from build123d import *

# Parameters (mm, degrees)
SKETCH1_W           = 12.7
SKETCH1_H           = 16.891
BOSS_EXTRUDE1_DEPTH = 3.175
SKETCH2_R           = 2.54
CUT_EXTRUDE1_DEPTH  = 4.175
SKETCH3_W           = 12.7
SKETCH3_H           = 3.175
BOSS_EXTRUDE2_DEPTH = 22.225
SKETCH4_R           = 2.54
CUT_EXTRUDE2_DEPTH  = 4.175
CUT_EXTRUDE3_DEPTH  = 4.175
CUT_EXTRUDE4_DEPTH  = 4.175


with BuildPart() as part:
    # Sketch1 → Boss-Extrude1 (new body)
    with BuildSketch(Plane(origin=(0, 0, 0), x_dir=(1, 0, 0), z_dir=(0, 1, 0))):
        with Locations((-16.427296288, 6.362973118)):
            Rectangle(SKETCH1_W, SKETCH1_H)
    extrude(amount=BOSS_EXTRUDE1_DEPTH)

    # Sketch2 → Cut-Extrude1 (cut, through all)
    with BuildSketch(Plane(origin=(0, 3.175, 0), x_dir=(1, 0, 0), z_dir=(0, 1, 0))):
        with Locations((-16.427296288, 5.537473118)):
            Circle(SKETCH2_R)
    extrude(amount=-CUT_EXTRUDE1_DEPTH, mode=Mode.SUBTRACT)

    # Sketch3 → Boss-Extrude2 (add)
    with BuildSketch(Plane.XZ):
        with Locations((-16.427296288, -13.220973118)):
            Rectangle(SKETCH3_W, SKETCH3_H)
    extrude(amount=BOSS_EXTRUDE2_DEPTH)

    # Sketch4 → Cut-Extrude2 (cut, through all)
    with BuildSketch(Plane.XY.offset(-11.633473118)):
        with Locations((-16.427296288, -14.605)):
            Circle(SKETCH4_R)
    extrude(amount=-CUT_EXTRUDE2_DEPTH, mode=Mode.SUBTRACT)

    # Sketch6 → Cut-Extrude3 (cut, through all)
    with BuildSketch(Plane.XY.offset(-11.633473118)):
        with BuildLine():
            Line((-10.077296288, -22.225), (-22.777296288, -22.225))
            Line((-22.777296288, -22.225), (-22.777296288, -18.739929724))
            ThreePointArc((-22.777296288, -18.739929724), (-16.427296288, -22.182608054), (-10.077296288, -18.739929724))
            Line((-10.077296288, -18.739929724), (-10.077296288, -22.225))
        make_face()
    extrude(amount=-CUT_EXTRUDE3_DEPTH, mode=Mode.SUBTRACT)

    # Sketch7 → Cut-Extrude4 (cut, through all)
    with BuildSketch(Plane.XZ):
        with BuildLine():
            Line((-22.777296288, -1.376737497), (-22.777296288, 2.082526882))
            Line((-22.777296288, 2.082526882), (-10.077296288, 2.082526882))
            Line((-10.077296288, 2.082526882), (-10.077296288, -1.376737497))
            ThreePointArc((-10.077296288, -1.376737497), (-16.427296288, 2.054247432), (-22.777296288, -1.376737497))
        make_face()
    extrude(amount=-CUT_EXTRUDE4_DEPTH, mode=Mode.SUBTRACT)


solid = part.part
Here's how the part is built. I have some questions about the finished solid (model axes, mm). A direction names the side the tool comes from. Coordinates: 2 decimals unless noted, no trailing zeros. Write each loop counter-clockwise with the first axis right and the second up, starting at its lowest first coordinate (ties: lowest second). Pieces come first, ordered by that corner, then holes.
Item 1: Will these pins go through, and if not, where does the flat tip stop? pin 1 (4 mm diameter, centred on x = -13.5, y = -6, fed in from +Z); pin 2 (4 mm diameter, centred on x = -19, z = -8, fed in from -Y).
Item 2: I want a section at C-C on z = -4.25. Write out the boundary of the cut face in (x, y) (3 decimals).
Item 3: On a 3-axis mill with a long thin cutter (end or side, diameter ignored), from which of +Z, -Z, +X, -X, +Y, -Y can I reach the whole of each face in a straight line? I mean faces 1 (the flat face through (-17, -11, -11.633)), 2 (the flat face through (-16.5, 3.175, -8.4)). Say none if no direction works.
Item 4: I want a section at A-A on x = -14.5. Write out the boundary of the cut face in (y, z) (3 decimals).
Item 5: If we mould it in two halves opening along X, with no side actions, what happens to faces 3 (the flat face through (-15, 0, -3)), 4 (the flat face through (-22.777, -5, -12)), 5 (the cylindrical face through (-18.44, 1.61, -3.99)), 6 (the cylindrical face through (-16.322, 1.565, 2.054))? For each: +X half, -X half, draft (parallel to the pull), parting line (faces both ways), or undercut.
Item 6: If I drill on line 1 (Z direction, x = -19, y = -5.25); line 2 (Y direction, x = -15.5, z = 1) (3 decimals); line 3 (Z direction, x = -17, y = 0.5), over which ranges is the centre line in solid material (lowest first)?
Item 7: I want a section at B-B on y = -13. Write out the boundary of the cut face in (x, z).
Item 8: I want a section at D-D on z = -9.75. Write out the boundary of the cut face in (x, y) (3 decimals), and give its area (3 significant figures).
Findings below:
1. pin 1: stops at z = -11.63
1. pin 2: stops at y = 0
2. outline: (-22.777, 0) - (-18.617, 0) - (-18.617, 3.175) - (-22.777, 3.175) - close; (-14.238, 0) - (-10.077, 0) - (-10.077, 3.175) - (-14.238, 3.175) - close
3. face 1: +Z, +X, -X, -Y
3. face 2: +Z, -Z, +X, -X, +Y
4. outline: (-21.933, -14.808) - (-16.259, -14.808) - (-16.259, -11.633) - (-21.933, -11.633) - close; (-12.951, -14.808) - (3.175, -14.808) - (3.175, -7.192) - (0, -7.192) - (0, -11.633) - (-12.951, -11.633) - close; (0, -3.883) - (3.175, -3.883) - (3.175, 1.806) - (0, 1.806) - close
5. face 3: draft
5. face 4: -X half
5. face 5: undercut
5. face 6: parting line
6. line 1: z = -14.81 to -11.63
6. line 2: y = 0 to 3.175
6. line 3: z = -14.81 to -8.01, -3.06 to 2.03
7. outline: (-22.78, -14.81) - (-18.4, -14.81) - (-18.4, -11.63) - (-22.78, -11.63) - close; (-14.46, -14.81) - (-10.08, -14.81) - (-10.08, -11.63) - (-14.46, -11.63) - close
8. outline: (-22.777, 0) - (-10.077, 0) - (-10.077, 3.175) - (-22.777, 3.175) - close
8. area: 40.3 mm2
